from build123d import *

# Parameters (mm, degrees)
F0_R     = 50
F1_DEPTH = 350
F2_W     = 140
F2_H     = 110
F2_R     = 50
F3_DEPTH = 200


# Not quite as in the source:
# - a feature names something its author has since deleted; it is built from what else it names


with BuildPart() as f1:
    # F0 (on Top) → F1 (new body)
    with BuildSketch(Plane.XY):
        Circle(F0_R)
    extrude(amount=F1_DEPTH)

    # F2 (on face) → F3 (join)
    with BuildSketch(Plane.XY.offset(350)):
        Rectangle(F2_W, F2_H)
        Circle(F2_R, mode=Mode.SUBTRACT)
        Circle(F2_R)
    extrude(amount=F3_DEPTH)


solid = f1.part
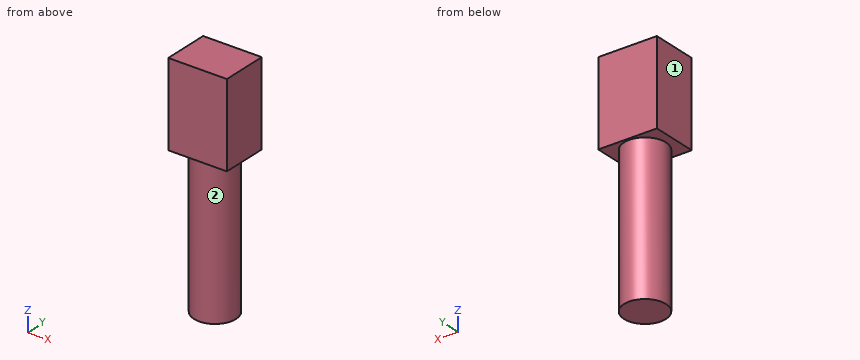
Work out the finished part from the listing and answer in its coordinate system (mm). Face numbers are marked on the shaded views. A direction names the side the tool comes from. Round coordinates to 2 decimals unless told otherwise and drop trailing zeros. Loops run counter-clockwise (first coordinate to the right, second up) from the corner with the lowest first, then second, coordinate; pieces in that order, holes last. Notation, with made-up numbers: (16, 70.25) - (38, 70.25) arc R27 ccw to (38, 104.25) - close; hole circle Ø8 at (-26, 51). An arc over 180 degrees is marked (long way). Use one line per item in the form item = value. Start each with the question number.
(1) Flat-ended cylindrical pins translate along their axes: P1, Ø10, axis at x = -3, z = 264, coming from the -Y side; P2, Ø8, axis at x = 18, z = 321.5, coming from the +Y side; P3, Ø5, axis at y = -19.5, z = 152, coming from the +X side. Find the tip coordinate at first contact, or state that the pin passes through.
(2) Which of the six approach directions +Z, -Z, +X, -X, +Y, -Y give full straight-line access (tool end or side, diameter ignored) to the marked faces 1 and 2?
(3) Consider line 1 (Z direction, x = -56, y = -10.5); line 2 (Y direction, x = -2, z = 318); line 3 (X direction, y = -0.5, z = 37). Determine where each line is inside the solid, lowest interval first.
(4) Find section A-A on x = 0. Determine the outline of the cut face in (y, z).
(5) Find section B-B on y = 0. Determine the outline of the cut face in (x, z).
(6) Find section C-C on z = 88.5. Determine the outline of the cut face in (x, y).
Answer list:
q1.P1 = -50
q1.P2 = 48
q1.P3 = 47.02
q2.face_1 = +Z, -Z, -X, +Y, -Y
q2.face_2 = -Z
q3.line_1 = 350 to 550
q3.line_2 = -49.96 to 49.96
q3.line_3 = -50 to 50
q4.outline = (-55, 350) - (-50, 350) - (-50, 0) - (50, 0) - (50, 350) - (55, 350) - (55, 550) - (-55, 550) - close
q5.outline = (-70, 350) - (-50, 350) - (-50, 0) - (50, 0) - (50, 350) - (70, 350) - (70, 550) - (-70, 550) - close
q6.outline = circle Ø100 at (0, 0)
